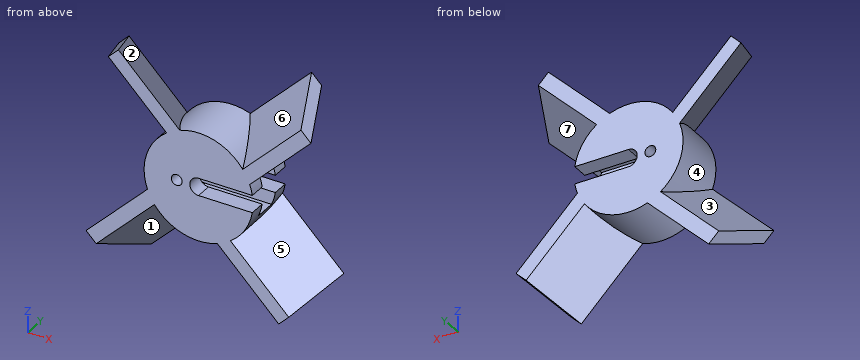
```python
from build123d import *

# Parameters (mm, degrees)
SKETCH1_R           = 10
BOSS_EXTRUDE1_DEPTH = 10
SKETCH3_R           = 1.6
CUT_EXTRUDE2_DEPTH  = 18.320508076
SKETCH7_W           = 3.2
SKETCH7_H           = 10
CUT_EXTRUDE6_DEPTH  = 10
SKETCH9_R           = 1
CUT_EXTRUDE7_DEPTH  = 18.320508076
SKETCH10_W          = 8
SKETCH10_H          = 4
CUT_EXTRUDE8_DEPTH  = 17
FILLET1_R           = 4
BOSS_EXTRUDE3_START = -0.920608418
BOSS_EXTRUDE3_DEPTH = 15.920608418
CIRPATTERN2_COUNT   = 4


# Read off the part's stored shape, not the designer's step: Boss-Extrude3
with BuildPart() as part:
    # Sketch1 → Boss-Extrude1 (new body)
    with BuildSketch(Plane(origin=(0, 0, 0), x_dir=(1, 0, 0), z_dir=(0, 1, 0))):
        with Locations(Location((0, 0, 0), (0, 0, 270))):
            Circle(SKETCH1_R)
    extrude(amount=BOSS_EXTRUDE1_DEPTH)

    # Sketch3 → Cut-Extrude2 (cut, through all)
    with BuildSketch(Plane(origin=(0, 10, 0), x_dir=(1, 0, 0), z_dir=(0, 1, 0))):
        with Locations(Location((0, 0, 0), (0, 0, 270))):
            Circle(SKETCH3_R)
    extrude(amount=-CUT_EXTRUDE2_DEPTH, mode=Mode.SUBTRACT)

    # Sketch7 → Cut-Extrude6 (cut)
    with BuildSketch(Plane(origin=(10, 0, 0), x_dir=(0, 0, -1), z_dir=(1, 0, 0))):
        with Locations((0, 5)):
            Rectangle(SKETCH7_W, SKETCH7_H)
    extrude(amount=-CUT_EXTRUDE6_DEPTH, mode=Mode.SUBTRACT)

    # Sketch9 → Cut-Extrude7 (cut, through all)
    with BuildSketch(Plane(origin=(0, 10, 0), x_dir=(1, 0, 0), z_dir=(0, 1, 0))):
        with Locations(Location((-4, 0, 0), (0, 0, 270))):
            Circle(SKETCH9_R)
    extrude(amount=-CUT_EXTRUDE7_DEPTH, mode=Mode.SUBTRACT)

    # Sketch10 → Cut-Extrude8 (cut)
    with BuildSketch(Plane(origin=(10, 0, 0), x_dir=(0, 0, -1), z_dir=(1, 0, 0))):
        with Locations((0, 5)):
            Rectangle(SKETCH10_W, SKETCH10_H)
    extrude(amount=-CUT_EXTRUDE8_DEPTH, mode=Mode.SUBTRACT)

    # Fillet1
    fillet1_edges = [part.edges().sort_by_distance(p)[0] for p in [
        (-7, 5, 4),
        (-7, 5, -4),
    ]]
    fillet(fillet1_edges, radius=FILLET1_R - 0.0001)  # a hair under: the kernel refuses the full size

    # Boss-Extrude3 outline → Boss-Extrude3 (add)
    with BuildSketch(Plane(origin=(7.071067812, 0, 7.071067812), x_dir=(0.7071067811865476, 0, -0.7071067811865476), z_dir=(0.7071067811865476, 0, 0.7071067811865476)).offset(BOSS_EXTRUDE3_START)):
        Polygon((4.191019983, 0), (-1.582482709, 10), (-4.191019983, 10), (1.582482709, 0), align=None)
    boss_extrude3 = extrude(amount=BOSS_EXTRUDE3_DEPTH)

    # CirPattern2: Boss-Extrude3 ×4 about axis
    cirpattern2_axis = Axis((0, 0, 0), (0, 1, 0))
    for i in range(1, CIRPATTERN2_COUNT):
        add(boss_extrude3.rotate(cirpattern2_axis, i * 360 / CIRPATTERN2_COUNT))


solid = part.part
```
Here's how the part is built. I have some questions about the finished solid (model axes, mm). Face numbers are marked on the shaded views. A direction names the side the tool comes from. Give positions to 0.01 mm unless a question says otherwise; leave off trailing zeros. Loops run counter-clockwise (first coordinate to the right, second up) from the corner with the lowest first, then second, coordinate; pieces in that order, holes last. Notation, with made-up numbers: M 15.25,24.5 L 29.25,24.5 A26 ccw 29.25,50.5 Z; hole C 39.5,-15.5 d9. An arc over 180 degrees is marked long. Put each result on its own line as item: value. Start each with the question number.
(1) Will these pins go through, and if not, where does the flat tip stop? pin 1 Ø1.6 at (x, z) = (-4, 0) entering from -Y; pin 2 Ø0.9 at (x, y) = (2.5, 8.5) entering from -Z; pin 3 Ø1 at (x, z) = (-10, 12) entering from +Y; pin 4 Ø2 at (x, z) = (-9, 13) entering from +Y.
(2) I want a section at A-A on z = -11.5. Please give me the cut outline in (x, y).
(3) I want a section at B-B on x = -1. Please give me the cut outline in (y, z).
(4) I want a section at C-C on z = 16. Please give me the cut outline in (x, y), then the cut area to 3 significant figures.
(5) For the marked faces 4, 5, 6 and 7, which set-ups out of +Z, -Z, +X, -X, +Y, -Y let a thin tool reach every point of the face, with its end or its side?
(6) If we mould it in two halves opening along Z, with no side actions, what happens to the marked faces 1, 2 and 3? For each: +Z half, -Z half, draft (parallel to the pull), parting line (faces both ways), or undercut.
(7) I need wall thicknesses on line 1 along X through (y, z) = (9.1, 0); line 2 along Z through (x, y) = (8, 5.5); line 3 along Z through (x, y) = (12.5, 7). Which ranges of each line are inside material? Lowest first, please. Write a range as [from, to].
Answer block:
1. pin 1: through
1. pin 2: z = -9.79
1. pin 3: y = 5.68
1. pin 4: y = 4.09
2. outline: M -17.43,0 L -13.74,0 L -5.57,10 L -9.26,10 Z; M 5.57,0 L 9.26,0 L 17.43,10 L 13.74,10 Z
3. outline: M 0,-9.95 L 10,-9.95 L 10,-1.25 L 7,-1.25 L 7,-4 L 3,-4 L 3,-1.25 L 0,-1.25 Z; M 0,1.25 L 3,1.25 L 3,4 L 7,4 L 7,1.25 L 10,1.25 L 10,9.95 L 0,9.95 Z
4. outline: M -19.36,6.85 L -13.76,0 L -10.07,0 L -18.24,10 L -19.36,10 Z; M 10.07,10 L 18.24,0 L 19.36,0 L 19.36,3.15 L 13.76,10 Z
4. area: 65.7 mm^2
5. face 4: -X
5. face 5: +X, -Y
5. face 6: +Z, -Y
5. face 7: +X, +Y
6. face 1: -Z half
6. face 2: +Z half
6. face 3: undercut
7. line 1: [-10, -5], [-3, -1.6]
7. line 2: [-9.44, -4], [4, 6], [6.56, 10.25]
7. line 3: [-12.71, -9.02], [12.29, 15.98]
